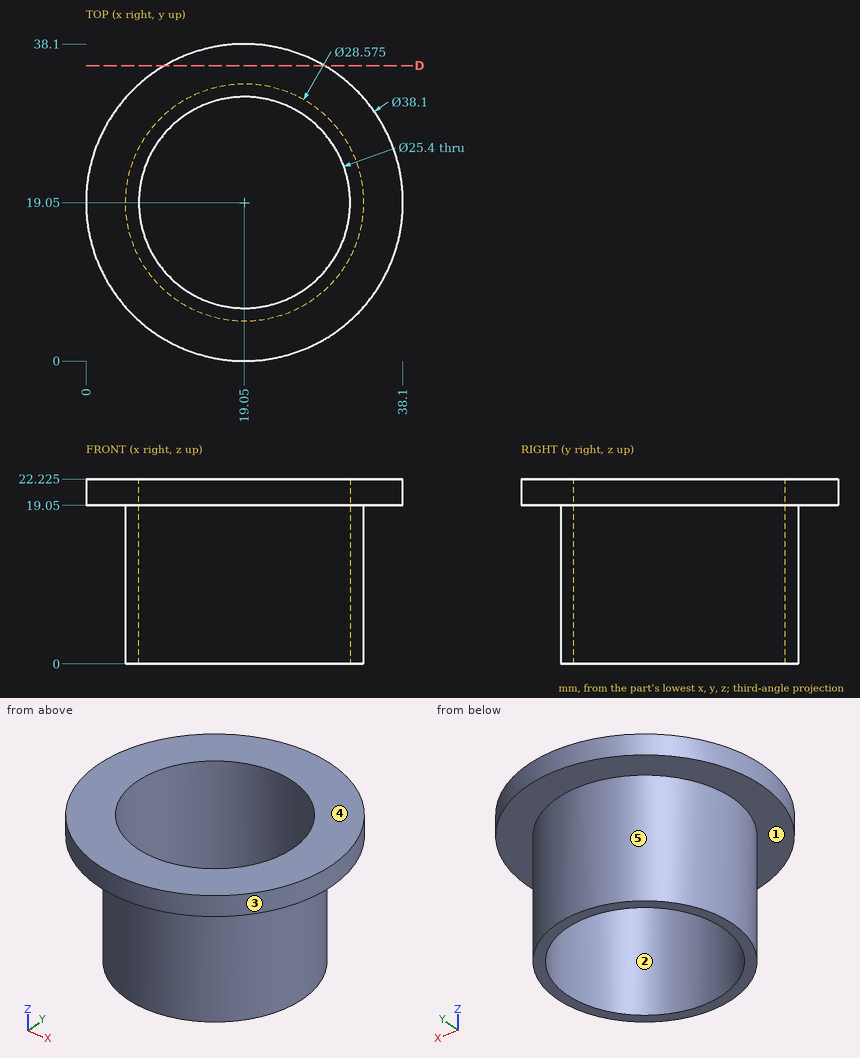
The drawing under review shows one solid part. Ordinate dimensions are in mm from its lowest x, y, z. A direction names the side the tool comes from. Round coordinates to 2 decimals unless told otherwise and drop trailing zeros. Order: outer loops, then holes, each group sorted by start corner. A loop starts at its lowest first (then second) coordinate and runs counter-clockwise, first axis right, second up. Notation, with made-up numbers: (-31.75, -17.75) - (8.25, -17.75) arc R28 ccw to (8.25, 10.25) - close; hole circle Ø9 at (60.25, -32). An arc over 180 degrees is marked (long way). Return JSON: item names as keys, results as strings.
Q1. The part is to be moulded in two halves that separate along Y. For the marked faces 1, 2 and 3, say which applies: pulls with the +Y half, pulls with the -Y half, needs draft (parallel to the pull), parting line crosses it, or undercut.
Computed values:
{"face 1": "needs draft", "face 2": "undercut", "face 3": "parting line crosses it"}
Q2. Consider section D-D on y = 35.5. Write out the cut boundary in (x, z) (3 decimals), plus the area to 3 significant figures.
Computed values:
{"outline": "(9.443, 19.05) - (28.657, 19.05) - (28.657, 22.225) - (9.443, 22.225) - close", "area": "61.0 mm2"}
Q3. For pin 1 Ø10 at (x, z) = (19, 7) entering from +Y; pin 2 Ø3 at (x, z) = (21, 20) entering from +Y; pin 3 Ø6 at (x, z) = (11, 17) entering from -Y; pin 4 Ø11.5 at (x, y) = (14.5, 23) entering from -Z, all flat-tipped, find the tip position at first contact; note any pin that passes through.
Computed values:
{"pin 1": "stops at y = 33.34", "pin 2": "stops at y = 38.09", "pin 3": "stops at y = 0.92", "pin 4": "passes through"}
Q4. Machinability: for the marked faces 4 and 5, which of the approach directions +Z, -Z, +X, -X, +Y, -Y give a long, thin tool a straight path to every point of the face, cutting with its end or side? Answer none if there is none.
Computed values:
{"face 4": "+Z, +X, -X, +Y, -Y", "face 5": "-Z"}
Q5. Wall thickness on L1, parallel to Y at x = 19.05, z = 16.75; L2, parallel to X at y = 19.5, z = 9.5; L3, parallel to X at y = 19.5, z = 20.25: over which ranges is each line inside the solid? List them lowest first. Write a range as [from, to].
Computed values:
{"L1": "y = [4.76, 6.35], [31.75, 33.34]", "L2": "x = [4.77, 6.36], [31.74, 33.33]", "L3": "x = [0.01, 6.36], [31.74, 38.09]"}
